The drawing under review shows one solid part. Ordinate dimensions are in mm from its lowest x, y, z. Round coordinates to 2 decimals unless told otherwise and drop trailing zeros. Write each loop counter-clockwise with the first axis right and the second up, starting at its lowest first coordinate (ties: lowest second). Pieces come first, ordered by that corner, then holes. Notation, with made-up numbers: (47.5, -22.75) -> (60.5, -22.75) arc R27 cw to (60.5, -0.75) -> close; hole circle Ø10 at (37, -36). An arc over 180 degrees is marked (long way). Answer in a Markdown table with one row per item. Add a question column.
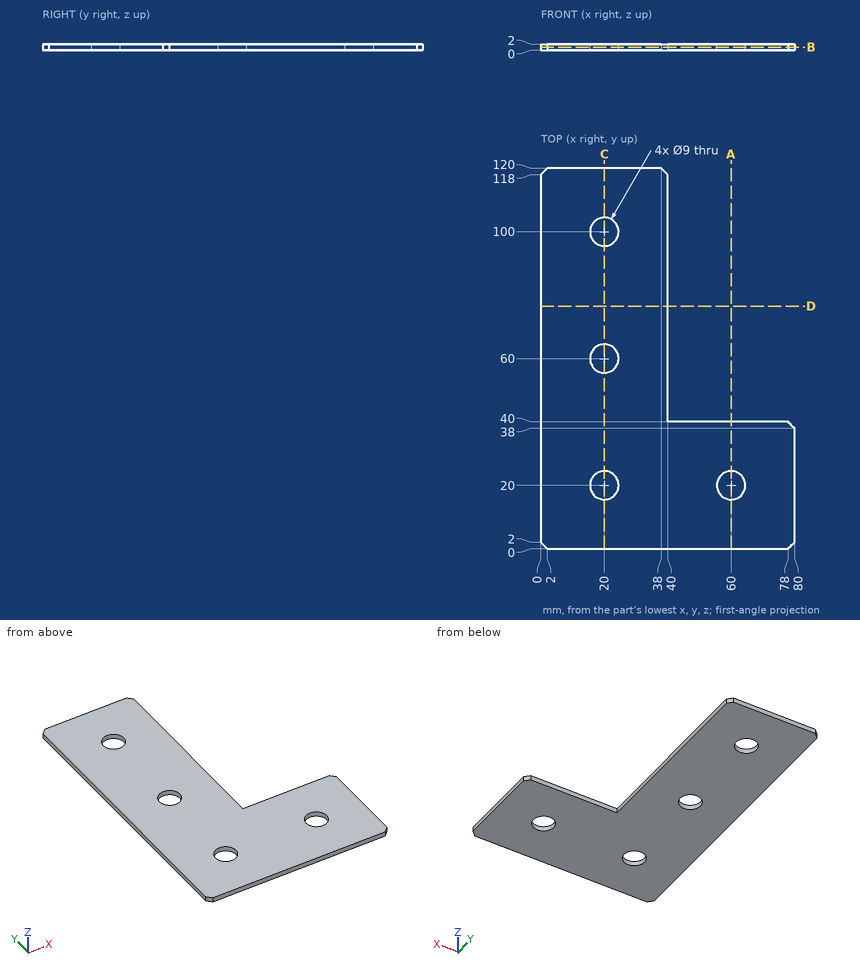
1. Insertion check: pin 1 Ø1 at (y, z) = (62.5, 1.5) entering from +X. The pin has a flat end and moves straight along its axis. Give the tip position at first contact, or say it passes through.
2. Add section D-D on y = 76.5. Write out the cut boundary in (x, z), plus the area to 3 significant figures.
3. Add section B-B on z = 1. Write out the cut boundary in (x, y).
4. For L1, parallel to Y at x = 20, z = 0.5; L2, parallel to X at y = 20, z = 0.7; L3, parallel to X at y = 23, z = 0.85, list the stretches that pass through material, from the lowest coordinate up.
5. Add section A-A on x = 60. Write out the cut boundary in (y, z).
6. Add section C-C on x = 20. Write out the cut boundary in (y, z), plus the area to 3 significant figures.
Filled in:
| question | item | result |
|---|---|---|
| 1 | pin 1 | x = 40 |
| 2 | outline | (0, 0) -> (40, 0) -> (40, 2) -> (0, 2) -> close |
| 2 | area | 80.0 mm² |
| 3 | outline | (0, 2) -> (2, 0) -> (78, 0) -> (80, 2) -> (80, 38) -> (78, 40) -> (40, 40) -> (40, 118) -> (38, 120) -> (2, 120) -> (0, 118) -> close; hole circle Ø9 at (20, 20); hole circle Ø9 at (20, 60); hole circle Ø9 at (20, 100); hole circle Ø9 at (60, 20) |
| 4 | L1 | 0 to 15.5, 24.5 to 55.5, 64.5 to 95.5, 104.5 to 120 |
| 4 | L2 | 0 to 15.5, 24.5 to 55.5, 64.5 to 80 |
| 4 | L3 | 0 to 16.65, 23.35 to 56.65, 63.35 to 80 |
| 5 | outline | (0, 0) -> (15.5, 0) -> (15.5, 2) -> (0, 2) -> close; (24.5, 0) -> (40, 0) -> (40, 2) -> (24.5, 2) -> close |
| 6 | outline | (0, 0) -> (15.5, 0) -> (15.5, 2) -> (0, 2) -> close; (24.5, 0) -> (55.5, 0) -> (55.5, 2) -> (24.5, 2) -> close; (64.5, 0) -> (95.5, 0) -> (95.5, 2) -> (64.5, 2) -> close; (104.5, 0) -> (120, 0) -> (120, 2) -> (104.5, 2) -> close |
| 6 | area | 186 mm² |
